The drawing under review shows one solid part. Ordinate dimensions are in mm from its lowest x, y, z. Round coordinates to 2 decimals unless told otherwise and drop trailing zeros. Write each loop counter-clockwise with the first axis right and the second up, starting at its lowest first coordinate (ties: lowest second). Pieces come first, ordered by that corner, then holes. Notation, with made-up numbers: M 34,-29.5 L 91,-29.5 A18 cw 91,-6.5 Z; hole C -8,61 d1. An arc over 180 degrees is marked long. One line per item, written item: value. Start each with the question number.
1) Wall thickness on probe 1 along X at (y, z) = (0.9, 39.5); probe 2 along X at (y, z) = (0.25, 61.5): over which ranges is each line inside the solid? List them lowest first.
2) Take a section at D-D, the plane y = 0.7. State how many separate pieces and enclosed holes the cut face has, and give its area (3 significant figures).
3) Take a section at C-C, the plane z = 60.5. Write out the cut boundary in (x, y) (1 decimal), and give its area (3 significant figures).
4) For P1, Ø1.5, axis at x = 41.5, y = 1, coming from the +Z side; P2, Ø1.8, axis at x = 39.5, z = 7, coming from the -Y side; P3, Ø1.5, axis at x = 10, y = 0.5, coming from the -Z side, all flat-tipped, find the tip position at first contact; note any pin that passes through.
5) Take a section at A-A, the plane x = 39.5. Write out the cut boundary in (y, z), and give its area (3 significant figures).
6) Take a section at B-B, the plane z = 32.5. Write out the cut boundary in (x, y) (1 decimal), and give its area (3 significant figures).
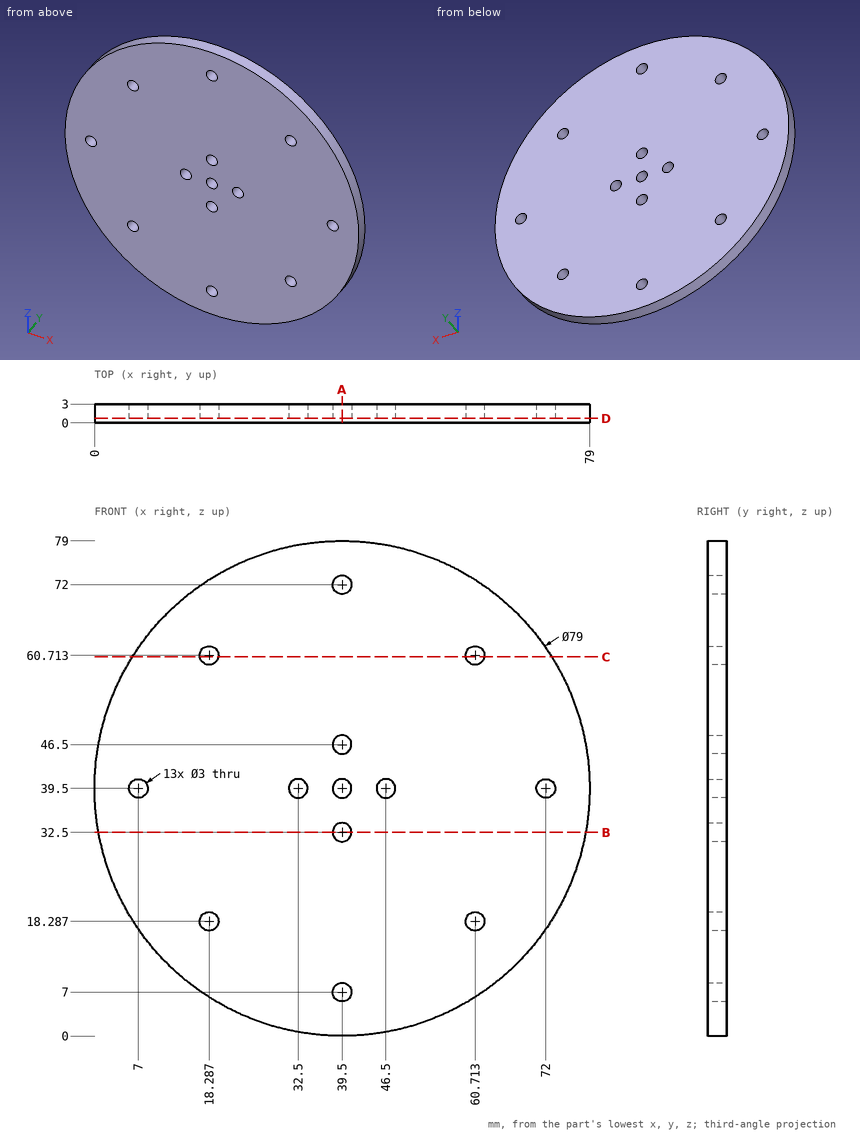
Checked values:
1. probe 1: x = 0 to 5.5, 8.5 to 31, 34 to 38, 41 to 45, 48 to 70.5, 73.5 to 79
1. probe 2: x = 6.69 to 17.01, 19.56 to 59.44, 61.99 to 72.31
2. separate pieces: 1
2. enclosed holes: 13
2. area: 4,810 mm2
3. outline: M 6,0 L 16.8,0 L 16.8,3 L 6,3 Z; M 19.8,0 L 59.2,0 L 59.2,3 L 19.8,3 Z; M 62.2,0 L 73,0 L 73,3 L 62.2,3 Z
3. area: 183 mm2
4. P1: stops at z = 78.98
4. P2: passes through
4. P3: stops at z = 12.41
5. outline: M 0,0 L 3,0 L 3,5.5 L 0,5.5 Z; M 0,8.5 L 3,8.5 L 3,31 L 0,31 Z; M 0,34 L 3,34 L 3,38 L 0,38 Z; M 0,41 L 3,41 L 3,45 L 0,45 Z; M 0,48 L 3,48 L 3,70.5 L 0,70.5 Z; M 0,73.5 L 3,73.5 L 3,79 L 0,79 Z
5. area: 192 mm2
6. outline: M 0.6,0 L 38,0 L 38,3 L 0.6,3 Z; M 41,0 L 78.4,0 L 78.4,3 L 41,3 Z
6. area: 224 mm2
